```python
from build123d import *

# Parameters (mm, degrees)
SKETCH1_W           = 42.6
SKETCH1_H           = 32.5
SKETCH1_R           = 1.4
SKETCH1_W_2         = 22.6
SKETCH1_H_2         = 12.5
BOSS_EXTRUDE1_DEPTH = 10


with BuildPart() as part:
    # Sketch1 → Boss-Extrude1 (new body)
    with BuildSketch(Plane(origin=(0, 0, 0), x_dir=(1, 0, 0), z_dir=(0, 1, 0))):
        Rectangle(SKETCH1_W, SKETCH1_H)
        with Locations(Location((-14.9, 0, 0), (0, 0, 270))):
            Circle(SKETCH1_R, mode=Mode.SUBTRACT)
        with Locations(Location((14.9, 0, 0), (0, 0, 90))):
            Circle(SKETCH1_R, mode=Mode.SUBTRACT)
        Rectangle(SKETCH1_W_2, SKETCH1_H_2, mode=Mode.SUBTRACT)
    extrude(amount=BOSS_EXTRUDE1_DEPTH)


solid = part.part
```
Verification items for the finished model (mm, model axes). A direction names the side the tool comes from. Coordinates: 2 decimals unless noted, no trailing zeros. Loops run counter-clockwise (first coordinate to the right, second up) from the corner with the lowest first, then second, coordinate; pieces in that order, holes last. Notation, with made-up numbers: (-6.75, 89.5) - (2.25, 89.5) arc R21 ccw to (2.25, 99.5) - close; hole circle Ø3 at (-30.75, -7). An arc over 180 degrees is marked (long way). Return JSON: item names as keys, results as strings.
1. Section check B-B, the plane z = 0. Record the boundary of the cut face in (x, y).
Established:
{"outline": "(-21.3, 0) - (-16.3, 0) - (-16.3, 10) - (-21.3, 10) - close; (-13.5, 0) - (-11.3, 0) - (-11.3, 10) - (-13.5, 10) - close; (11.3, 0) - (13.5, 0) - (13.5, 10) - (11.3, 10) - close; (16.3, 0) - (21.3, 0) - (21.3, 10) - (16.3, 10) - close"}
2. Mould release check, pull along X, two halves, no side actions. Record for faces 1 (the flat face through (-11.3, 5, 0)), 2 (the flat face through (0, 0, -7)), 3 (the flat face through (-21.3, 5, 0)): +X half, -X half, draft (parallel to the pull), parting line (faces both ways), or undercut.
Established:
{"face 1": "undercut", "face 2": "draft", "face 3": "-X half"}
3. Thickness scan on L1, parallel to X at y = 7.75, z = 0; L2, parallel to X at y = 6.5, z = 1.5; L3, parallel to Z at x = -8.5, y = 6.75. Record the ranges inside material, lowest first.
Established:
{"L1": "x = -21.3 to -16.3, -13.5 to -11.3, 11.3 to 13.5, 16.3 to 21.3", "L2": "x = -21.3 to -11.3, 11.3 to 21.3", "L3": "z = -16.25 to -6.25, 6.25 to 16.25"}
4. Section check A-A, the plane x = 14.9. Record the boundary of the cut face in (y, z).
Established:
{"outline": "(0, -16.25) - (10, -16.25) - (10, -1.4) - (0, -1.4) - close; (0, 1.4) - (10, 1.4) - (10, 16.25) - (0, 16.25) - close"}
5. Section check D-D, the plane x = -5. Record the boundary of the cut face in (y, z).
Established:
{"outline": "(0, -16.25) - (10, -16.25) - (10, -6.25) - (0, -6.25) - close; (0, 6.25) - (10, 6.25) - (10, 16.25) - (0, 16.25) - close"}
6. Tool access check on faces 4 (the flat face through (0, 5, 6.25)), 5 (the flat face through (21.3, 5, 0)). Record the directions out of +Z, -Z, +X, -X, +Y, -Y that give a thin tool (end or side, any length) a straight path to the whole face; none if there is none.
Established:
{"face 4": "+Y, -Y", "face 5": "+Z, -Z, +X, +Y, -Y"}
7. Section check C-C, the plane y = 8.75. Record the boundary of the cut face in (x, z).
Established:
{"outline": "(-21.3, -16.25) - (21.3, -16.25) - (21.3, 16.25) - (-21.3, 16.25) - close; hole circle Ø2.8 at (-14.9, 0); hole (-11.3, -6.25) - (11.3, -6.25) - (11.3, 6.25) - (-11.3, 6.25) - close; hole circle Ø2.8 at (14.9, 0)"}
